CAD build for the part. Positions are in the model's coordinates, mm. A direction names the side the tool comes from. Give positions to 0.01 mm unless a question says otherwise; leave off trailing zeros. Write each loop counter-clockwise with the first axis right and the second up, starting at its lowest first coordinate (ties: lowest second). Pieces come first, ordered by that corner, then holes. Notation, with made-up numbers: (46, -23) - (87, -23) arc R35 ccw to (87, 16) - close; hole circle Ø4 at (57.5, 34). An arc over 180 degrees is marked (long way). Put each result on its own line as item: value. Start each with the question number.
1. Mould opens along X. For faces 4 (the flat face through (-25, 0, 5)), 5 (the flat face through (25, 0, 5)), 6 (the flat face through (20, 0, 0)), 7 (the flat face through (0, -14, 20)) say: +X half, -X half, draft (parallel to the pull), parting line (faces both ways), or undercut.
2. Cut at A-A on y = -15.5. List the corners of the cut face in (x, z).
3. Tool access for faces 1 (the flat face through (0, 0, 40.4)), 2 (the flat face through (-23, 0, -10)), 3 (the flat face through (-20, 0, 0)): list every direction of +Z, -Z, +X, -X, +Y, -Y with a clear straight run to the whole face (end or side of a thin tool).
4. Cut at B-B on x = 0. List the corners of the cut face in (y, z).
5. Wall check: line 1 (Y direction, x = 0, z = 48); line 2 (X direction, y = -17, z = 7.5). Give the ranges that are in metal, low to high.
6. Cut at D-D on y = 0. List the corners of the cut face in (x, z).
7. Cut at C-C on z = 48. List the corners of the cut face in (x, y).
8. Drop flat-ended pins along their axis: pin 1 (3 mm diameter, centred on y = 12.5, z = 44.5, fed in from +X); pin 2 (10 mm diameter, centred on x = 9.5, y = 9.5, fed in from -Z); pin 3 (15 mm diameter, centred on x = 0, y = 0, fed in from +Z). Give the stop position or say it passes through.
Autodesk Inventor part; units mm, degrees
ref_plane "YZ Plane" through (0, 0, 0) normal (1, 0, 0) x (0, 1, 0)
ref_plane "XZ Plane" through (0, 0, 0) normal (0, 1, 0) x (-1, 0, 0)
ref_plane "XY Plane" through (0, 0, 0) normal (0, 0, 1) x (1, 0, 0)
sketch "Sketch1" plane through (0, 0, 0) normal (0, 1, 0) x (-1, 0, 0)
  line L0 (20, 0) -> (20, 20)
  line L1 (20, 20) -> (-20, 20)
  line L2 (-20, 20) -> (-20, 0)
  line L3 (20, 10) -> (-20, 10)
  dimension "d49" = 40
extrude "Extrusion1" add sketch "Sketch1" along normal mid plane 40
sketch "Sketch6" plane through (0, 0, 0) normal (0, 0, 1) x (1, 0, 0)
  circle A0 centre (0, 0) radius 12.7
  dimension "d33" = 25.4
extrude "Extrusion6" add sketch "Sketch6" along normal blind 55.4
hole "Hole2" at (0, 0, 55.4) direction (0, 0, -1) diameter 19 depth 15
fillet "Fillet3" radius 1 1 edges at (-12.7, 0, 55.4)
sketch "Sketch8" plane through (0, 0, 0) normal (0, 0, -1) x (-1, 0, 0)
  circle A0 centre (0, 0) radius 13
extrude "Extrusion8" cut sketch "Sketch8" against normal blind 10
sketch "Sketch10" plane through (-20, 20, 20) normal (0, 0, 1) x (1, 0, 0)
  line L0 (0, 0) -> (-5, 0)
  line L1 (-5, 0) -> (-5, -40)
  line L2 (-5, -40) -> (0, -40)
  line L3 (0, -40) -> (0, 0)
  line L4 (40, 0) -> (45, 0)
  line L5 (45, 0) -> (45, -40)
  line L6 (45, -40) -> (40, -40)
  line L7 (40, -40) -> (40, 0)
  point P0 (20, -20)
extrude "Extrusion9" add sketch "Sketch10" against normal blind 30
properties part number "suporte-barra" material "Steel, Carbon"
Report:
1. face 4: -X half
1. face 5: +X half
1. face 6: undercut
1. face 7: draft
2. outline: (-25, -10) - (-20, -10) - (-20, 10) - (20, 10) - (20, -10) - (25, -10) - (25, 20) - (-25, 20) - close
3. face 1: +Z
3. face 2: -Z, +X, -X, +Y, -Y
3. face 3: -Z, +Y, -Y
4. outline: (-20, 10) - (20, 10) - (20, 20) - (12.7, 20) - (12.7, 54.4) arc R1 ccw to (11.7, 55.4) - (9.5, 55.4) - (9.5, 40.4) - (-9.5, 40.4) - (-9.5, 55.4) - (-11.7, 55.4) arc R1 ccw to (-12.7, 54.4) - (-12.7, 20) - (-20, 20) - close
5. line 1: y = -12.7 to -9.5, 9.5 to 12.7
5. line 2: x = -25 to -20, 20 to 25
6. outline: (-25, -10) - (-20, -10) - (-20, 10) - (20, 10) - (20, -10) - (25, -10) - (25, 20) - (12.7, 20) - (12.7, 54.4) arc R1 ccw to (11.7, 55.4) - (9.5, 55.4) - (9.5, 40.4) - (-9.5, 40.4) - (-9.5, 55.4) - (-11.7, 55.4) arc R1 ccw to (-12.7, 54.4) - (-12.7, 20) - (-25, 20) - close
7. outline: circle Ø25.4 at (0, 0); hole circle Ø19 at (0, 0)
8. pin 1: stops at x = 6.35
8. pin 2: stops at z = 10
8. pin 3: stops at z = 40.4
